Answer from the drawing. Dimensions are ordinates in mm from the lowest x, y and z of the part. A direction names the side the tool comes from. Round coordinates to 2 decimals unless told otherwise and drop trailing zeros. Loops run counter-clockwise (first coordinate to the right, second up) from the corner with the lowest first, then second, coordinate; pieces in that order, holes last. Notation, with made-up numbers: (-36, -16.5) - (-5, -16.5) arc R19 ccw to (-5, -12.5) - close; hole circle Ø6 at (87, 22). An arc over 180 degrees is marked (long way). Write item = value, one per line. Start each with the question number.
1) Section D-D, the plane x = 63.5 is taken. Determine the outline of the cut face in (y, z).
2) Given pin 1 Ø6 at (x, z) = (20.5, 15) entering from -Y; pin 2 Ø1 at (x, y) = (48, 3) entering from +Z; pin 3 Ø1.9 at (y, z) = (3.5, 42.5) entering from +X, each flat-ended and moving along its own axis, determine where each tip first touches the part or whether it passes through.
3) Section B-B, the plane x = 12.7 is taken. Determine the outline of the cut face in (y, z).
4) A tool of negligible diameter and unlimited length cuts with its end or side. For the marked faces 1 and 2, from which of +Z, -Z, +X, -X, +Y, -Y can it reach the whole face along a straight path? Write none if from no direction.
5) Section A-A, the plane z = 12.7 is taken. Determine the outline of the cut face in (x, y), and give its area (3 significant figures).
6) Section C-C, the plane y = 4.25 is taken. Determine the outline of the cut face in (x, z), and give its area (3 significant figures).
7) Straight lines are drawn through the part: line 1 along Z through (x, y) = (12.7, 5); line 2 along X through (y, z) = (3, 12.7); line 3 along Z through (x, y) = (50.8, 3). For each, find the intervals that lie inside material, in ascending order.
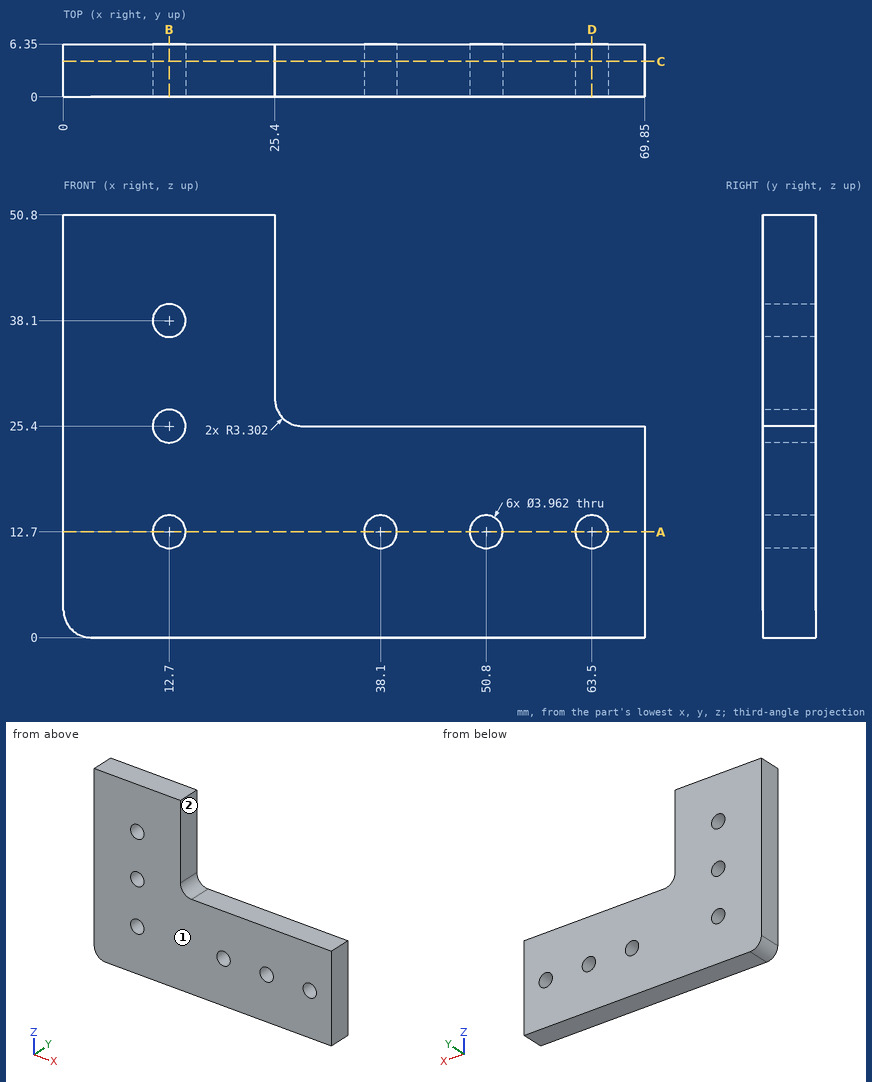
Geometry check:
q1.outline = (0, 0) - (6.35, 0) - (6.35, 10.72) - (0, 10.72) - close; (0, 14.68) - (6.35, 14.68) - (6.35, 25.4) - (0, 25.4) - close
q2.pin_1 = 0
q2.pin_2 = 25.4
q2.pin_3 = 25.4
q3.outline = (0, 0) - (6.35, 0) - (6.35, 10.72) - (0, 10.72) - close; (0, 14.68) - (6.35, 14.68) - (6.35, 23.42) - (0, 23.42) - close; (0, 27.38) - (6.35, 27.38) - (6.35, 36.12) - (0, 36.12) - close; (0, 40.08) - (6.35, 40.08) - (6.35, 50.8) - (0, 50.8) - close
q4.face_1 = +Z, -Z, +X, -X, -Y
q4.face_2 = +Z, +X, +Y, -Y
q5.outline = (0, 0) - (10.72, 0) - (10.72, 6.35) - (0, 6.35) - close; (14.68, 0) - (36.12, 0) - (36.12, 6.35) - (14.68, 6.35) - close; (40.08, 0) - (48.82, 0) - (48.82, 6.35) - (40.08, 6.35) - close; (52.78, 0) - (61.52, 0) - (61.52, 6.35) - (52.78, 6.35) - close; (65.48, 0) - (69.85, 0) - (69.85, 6.35) - (65.48, 6.35) - close
q5.area = 343 mm2
q6.outline = (0, 3.3) arc R3.3 ccw to (3.3, 0) - (69.85, 0) - (69.85, 25.4) - (28.7, 25.4) arc R3.3 cw to (25.4, 28.7) - (25.4, 50.8) - (0, 50.8) - close; hole circle Ø3.96 at (12.7, 12.7); hole circle Ø3.96 at (12.7, 25.4); hole circle Ø3.96 at (12.7, 38.1); hole circle Ø3.96 at (38.1, 12.7); hole circle Ø3.96 at (50.8, 12.7); hole circle Ø3.96 at (63.5, 12.7)
q6.area = 2,350 mm2
q7.line_1 = 0 to 10.72, 14.68 to 23.42, 27.38 to 36.12, 40.08 to 50.8
q7.line_2 = 0 to 10.72, 14.68 to 36.12, 40.08 to 48.82, 52.78 to 61.52, 65.48 to 69.85
q7.line_3 = 0 to 10.72, 14.68 to 25.4
